Design review of the part shown in the three views and the two pictorial views. Dimensions are in mm from the part's minimum x, y and z. A direction names the side the tool comes from. Give positions to 0.01 mm unless a question says otherwise; leave off trailing zeros. Write each loop counter-clockwise with the first axis right and the second up, starting at its lowest first coordinate (ties: lowest second). Pieces come first, ordered by that corner, then holes.
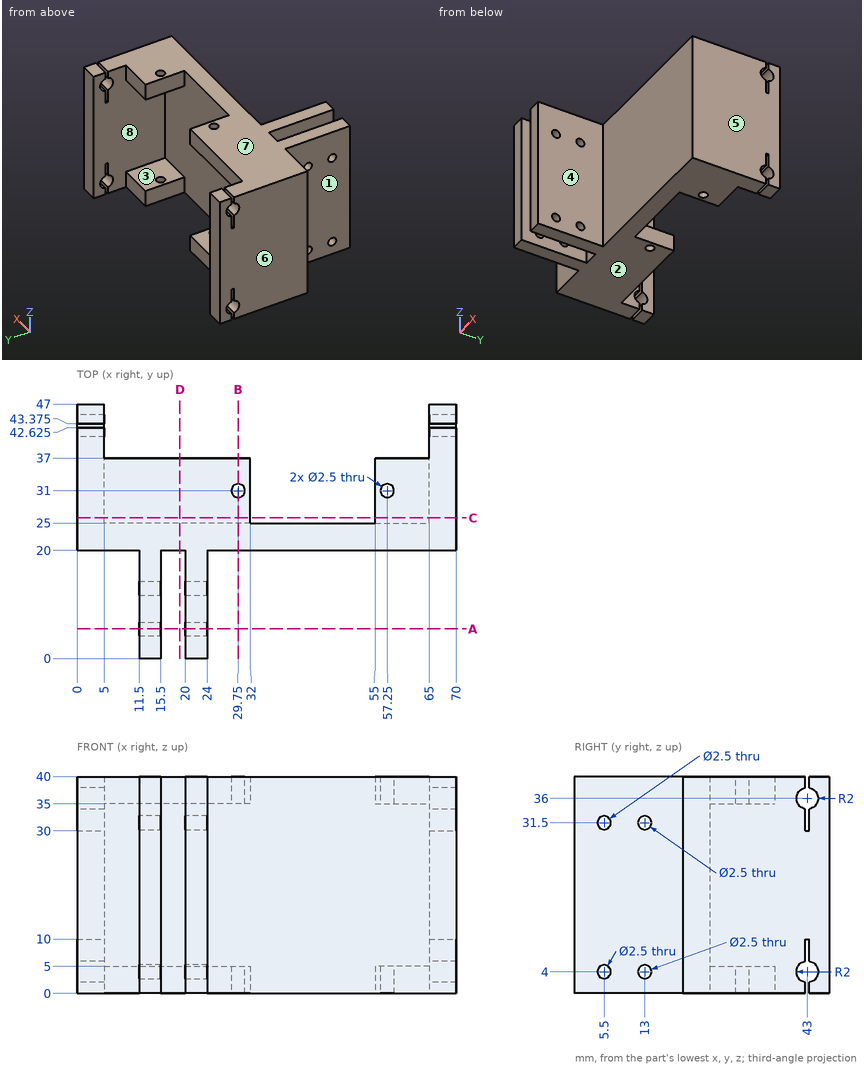
(1) Consider section B-B, the plane x = 29.75. Give the boundary of the cut face in (y, z).
Resolved:
outline: (20, 0) - (29.75, 0) - (29.75, 5) - (25, 5) - (25, 35) - (29.75, 35) - (29.75, 40) - (20, 40) - close; (32.25, 0) - (37, 0) - (37, 5) - (32.25, 5) - close; (32.25, 35) - (37, 35) - (37, 40) - (32.25, 40) - close
(2) Mouldability with a two-part tool opening along X and no side actions: class the marked faces 5, 6, 7 and 8 as pulls with the +X half, pulls with the -X half, needs draft (parallel to the pull), parting line crosses it, or undercut.
Resolved:
face 5: pulls with the +X half
face 6: pulls with the -X half
face 7: needs draft
face 8: undercut
(3) Clearance check with flat-ended pins moving along their axes: P1, Ø3.5, axis at x = 17, z = 15.5, coming from the -Y side; P2, Ø8, axis at x = 46, z = 35, coming from the -Y side; P3, Ø2, axis at x = 29.75, y = 31, coming from the +Z side; P4, Ø4, axis at x = 23.5, z = 2, coming from the +Y side. State where each tip first meets the part, or that it passes through.
Resolved:
P1: stops at y = 0
P2: stops at y = 20
P3: passes through
P4: stops at y = 37
(4) Consider section C-C, the plane y = 26. Give the boundary of the cut face in (x, z), then the cut area to 3 significant figures.
Resolved:
outline: (0, 0) - (32, 0) - (32, 5) - (5, 5) - (5, 35) - (32, 35) - (32, 40) - (0, 40) - close; (55, 0) - (70, 0) - (70, 40) - (55, 40) - (55, 35) - (65, 35) - (65, 5) - (55, 5) - close
area: 770 mm2
(5) Consider section D-D, the plane x = 19. Give the boundary of the cut face in (y, z), then the cut area to 3 significant figures.
Resolved:
outline: (20, 0) - (37, 0) - (37, 5) - (25, 5) - (25, 35) - (37, 35) - (37, 40) - (20, 40) - close
area: 320 mm2
(6) To check wall thickness, follow L1, parallel to Y at x = 13.75, z = 31.5; L2, parallel to X at y = 31, z = 36.45; L3, parallel to Z at x = 23, y = 13. State the ranges of each line that lie inside material, in increasing order.
Resolved:
L1: y = 0 to 4.25, 6.75 to 11.75, 14.25 to 25
L2: x = 0 to 28.5, 31 to 32, 55 to 56, 58.5 to 70
L3: z = 0 to 2.75, 5.25 to 30.25, 32.75 to 40
(7) Tool access review of the marked faces 1, 2, 3 and 4: name each direction out of +Z, -Z, +X, -X, +Y, -Y from which nothing blocks a thin tool from reaching the whole face with its end or side.
Resolved:
face 1: +Z, -Z, -X, -Y
face 2: -Z, +X, -X, +Y, -Y
face 3: +Y
face 4: +Z, -Z, +X, -Y
(8) Consider section A-A, the plane y = 5.5. Give the boundary of the cut face in (x, z), then the cut area to 3 significant figures.
Resolved:
outline: (11.5, 0) - (15.5, 0) - (15.5, 2.75) - (11.5, 2.75) - close; (11.5, 5.25) - (15.5, 5.25) - (15.5, 30.25) - (11.5, 30.25) - close; (11.5, 32.75) - (15.5, 32.75) - (15.5, 40) - (11.5, 40) - close; (20, 0) - (24, 0) - (24, 2.75) - (20, 2.75) - close; (20, 5.25) - (24, 5.25) - (24, 30.25) - (20, 30.25) - close; (20, 32.75) - (24, 32.75) - (24, 40) - (20, 40) - close
area: 280 mm2
